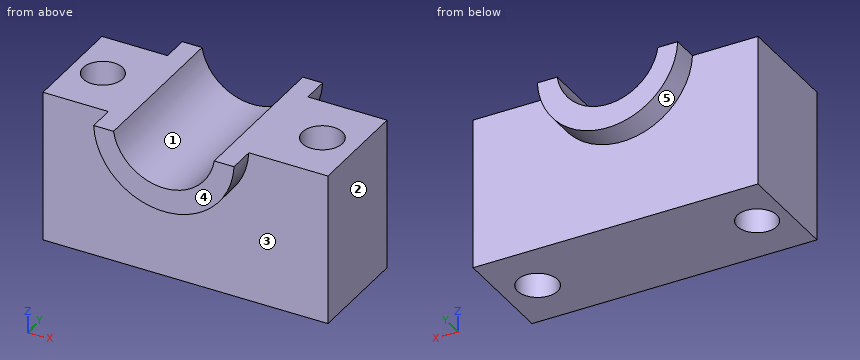
from build123d import *

# Parameters (mm, degrees)
F0_W          = 136.6302669048
F0_H          = 117.5191476941
F1_DEPTH      = 25.4
F1_DEPTH_BACK = 25.4
F2_R          = 33.6837672498
F3_DEPTH      = 38.1
F3_DEPTH_BACK = 38.1
F4_R          = 24.4259968854
F5_DEPTH      = 38.101
F5_DEPTH_BACK = 38.101
F6_W          = 151.7480313778
F6_H          = 49.3466332555
F7_DEPTH      = 38.101
F7_DEPTH_BACK = 38.101
F8_R          = 9.4700300279
F8_R_2        = 9.6065127636
F9_DEPTH      = 56.6212700138
F9_DEPTH_BACK = 16.1170975695


with BuildPart() as f1:
    # F0 (on Front) → F1 (new body, two sides)
    with BuildSketch(Plane.XZ) as f1_sk:
        with Locations((3.2802671194, 2.1393038332)):
            Rectangle(F0_W, F0_H)
    extrude(amount=F1_DEPTH)
    extrude(f1_sk.sketch, amount=-F1_DEPTH_BACK)

    # F2 (on Front) → F3 (join, two sides)
    with BuildSketch(Plane.XZ) as f3_sk:
        with Locations((0, 17.5422988832)):
            Circle(F2_R)
    extrude(amount=F3_DEPTH)
    extrude(f3_sk.sketch, amount=-F3_DEPTH_BACK)

    # F4 (on Front) → F5 (cut, two sides)
    with BuildSketch(Plane.XZ) as f5_sk:
        with Locations((0, 19.8242235929)):
            Circle(F4_R)
    extrude(amount=-F5_DEPTH, mode=Mode.SUBTRACT)
    extrude(f5_sk.sketch, amount=F5_DEPTH_BACK, mode=Mode.SUBTRACT)

    # F6 (on Front) → F7 (cut, two sides)
    with BuildSketch(Plane.XZ) as f7_sk:
        with Locations((0, 40.7894141972)):
            Rectangle(F6_W, F6_H)
    extrude(amount=-F7_DEPTH, mode=Mode.SUBTRACT)
    extrude(f7_sk.sketch, amount=F7_DEPTH_BACK, mode=Mode.SUBTRACT)

    # F8 (on Top) → F9 (cut, two sides)
    with BuildSketch(Plane.XY) as f9_sk:
        with Locations((-50.4875965416, 0)):
            Circle(F8_R)
        with Locations((54.7662004828, 0)):
            Circle(F8_R_2)
    extrude(amount=-F9_DEPTH, mode=Mode.SUBTRACT)
    extrude(f9_sk.sketch, amount=F9_DEPTH_BACK, mode=Mode.SUBTRACT)


solid = f1.part
Could you check a few things on this model? Use its own coordinates, in mm. Face numbers are marked on the shaded views. A direction names the side the tool comes from. Round coordinates to 2 decimals unless told otherwise and drop trailing zeros. Write each loop counter-clockwise with the first axis right and the second up, starting at its lowest first coordinate (ties: lowest second). Pieces come first, ordered by that corner, then holes. Notation, with made-up numbers: (-21, -38) - (1, -38) arc R24 ccw to (1, -22) - close; hole circle Ø4 at (80.25, 27). An arc over 180 degrees is marked (long way). Put each result on its own line as item: value. Start each with the question number.
(1) I want a section at A-A, the plane y = 0. Please give me the cut outline in (x, z).
(2) I want a section at B-B, the plane z = -10.5. Please give me the cut outline in (x, y).
(3) Thinking about a two-plate mould opening in X: for the marked faces 1, 2 and 3, which applies, released by +X, released by -X, zero draft, split by the parting line, or undercut?
(4) I want a section at D-D, the plane x = 0. Please give me the cut outline in (y, z), plus the area to 3 significant figures.
(5) For the marked faces 4 and 5, which set-ups out of +Z, -Z, +X, -X, +Y, -Y let a thin tool reach every point of the face, with its end or its side?
(6) I want a section at C-C, the plane x = 57. Please give me the cut outline in (y, z).
(7) Will these pins go through, and if not, where does the flat tip stop? pin 1 (17 mm diameter, centred on x = -50.49, y = 0, fed in from -Z); pin 2 (1.5 mm diameter, centred on x = 38.5, z = 8.5, fed in from -Y); pin 3 (12 mm diameter, centred on x = -6.5, y = 2, fed in from +Z).
(8) I need wall thicknesses on probe 1 along X at (y, z) = (-1, -35); probe 2 along X at (y, z) = (0, 4.75); probe 3 along X at (y, z) = (6, 4). Which ranges of each line are inside material? Lowest first, please.
Here are the results:
1. outline: (-65.03, -56.62) - (-59.96, -56.62) - (-59.96, 16.12) - (-65.03, 16.12) - close; (-41.02, -56.62) - (45.16, -56.62) - (45.16, 16.12) - (24.14, 16.12) arc R24.43 cw to (-24.14, 16.12) - (-41.02, 16.12) - close; (64.37, -56.62) - (71.6, -56.62) - (71.6, 16.12) - (64.37, 16.12) - close
2. outline: (-65.03, -25.4) - (-18.66, -25.4) - (-18.66, -38.1) - (18.66, -38.1) - (18.66, -25.4) - (71.6, -25.4) - (71.6, 25.4) - (18.66, 25.4) - (18.66, 38.1) - (-18.66, 38.1) - (-18.66, 25.4) - (-65.03, 25.4) - close; hole circle Ø18.94 at (-50.49, 0); hole circle Ø19.21 at (54.77, 0)
3. face 1: undercut
3. face 2: released by +X
3. face 3: zero draft
4. outline: (-38.1, -16.14) - (-25.4, -16.14) - (-25.4, -56.62) - (25.4, -56.62) - (25.4, -16.14) - (38.1, -16.14) - (38.1, -4.6) - (-38.1, -4.6) - close
4. area: 2,940 mm^2
5. face 4: +Z, -Z, +X, -X, -Y
5. face 5: -Z, +Y
6. outline: (-25.4, -56.62) - (-9.34, -56.62) - (-9.34, 16.12) - (-25.4, 16.12) - close; (9.34, -56.62) - (25.4, -56.62) - (25.4, 16.12) - (9.34, 16.12) - close
7. pin 1: passes through
7. pin 2: stops at y = -25.4
7. pin 3: stops at z = -1.16
8. probe 1: x = -65.03 to -59.9, -41.07 to 45.21, 64.32 to 71.6
8. probe 2: x = -65.03 to -59.96, -41.02 to -19.22, 19.22 to 45.16, 64.37 to 71.6
8. probe 3: x = -65.03 to -57.81, -43.16 to -18.61, 18.61 to 47.26, 62.27 to 71.6
